Verification items for the finished model (mm, model axes). A direction names the side the tool comes from. Give positions to 0.01 mm unless a question says otherwise; leave off trailing zeros. Order: outer loops, then holes, each group sorted by start corner. A loop starts at its lowest first (then second) coordinate and runs counter-clockwise, first axis right, second up. Notation, with made-up numbers: (82.5, -38) -> (131.5, -38) arc R36 cw to (131.5, -4) -> close; hole circle Ø8 at (-38, 87). An arc over 180 degrees is marked (long way). Return JSON: item names as keys, results as strings. Group by question number.
(1) Cross-section at C-C on z = 4. Enter the section's corners in (x, y), then the cut area to 3 significant figures.
(2) Cross-section at A-A on z = 0. Enter the section's corners in (x, y) (1 decimal).
(3) Depth check by flat-ended pin: pin 1 Ø8.5 at (x, z) = (0, 14.225) entering from +Y; pin 2 Ø6 at (x, y) = (-10, 12) entering from +Z; pin 3 Ø6 at (y, z) = (24, -13.5) entering from -X; pin 4 Ø8 at (y, z) = (4, 10) entering from -X. Enter the tip coordinate at first touch or a pass-through.
(4) Cross-section at D-D on y = 23.5. Enter the section's corners in (x, z) (1 decimal).
(5) Thickness scan on line 1 along Z through (x, y) = (0, 13) (1 decimal); line 2 along X through (y, z) = (20.5, -2); line 3 along Y through (x, z) = (-4.5, 16.5). Record the ranges inside material, lowest first.
(6) Release check for a two-part mould opening along Z. For faces 1 (the face through (6.633, 27.126, -6.083)), 2 (the face through (4, 0, 4)), 3 (the face through (-0.559, 8.874, 11.706)) record: pulls with the +Z half, pulls with the -Z half, needs draft (parallel to the pull), parting line crosses it, or undercut.
(7) Cross-section at B-B on x = 0. Enter the section's corners in (y, z) (1 decimal), then the cut area to 3 significant figures.
(8) Tool access check on faces 4 (the face through (-0.559, 8.874, -16.744)), 5 (the face through (-8.2, 18, -4.5)). Record the directions out of +Z, -Z, +X, -X, +Y, -Y that give a thin tool (end or side, any length) a straight path to the whole face; none if there is none.
from build123d import *

# Parameters (mm, degrees)
CUT_EXTRUDE1_REACH = 46.922
SKETCH2_R          = 4.7625
SKETCH3_R          = 2.58
CUT_EXTRUDE2_DEPTH = 45.92215489


with BuildPart() as part:
    # Sketch1 → Revolve1 (revolve)
    with BuildSketch(Plane.XY, mode=Mode.PRIVATE) as revolve1_sk:
        Polygon((0, 0), (19, 0), (19, 18), (9, 18), (9, 36), (0, 36), align=None)
    revolve(revolve1_sk.sketch.rotate(Axis((0, 36, 0), (0, -1, 0)), 180), axis=Axis((0, 36, 0), (0, -1, 0)))

    # Sketch2 → Cut-Extrude1 (cut, up to next)
    with BuildSketch(Plane.XZ, mode=Mode.PRIVATE) as cut_extrude1_sk1:
        Circle(SKETCH2_R)
    cut_extrude1_tool1 = extrude(cut_extrude1_sk1.sketch, amount=-CUT_EXTRUDE1_REACH, mode=Mode.PRIVATE) & part.part
    add(cut_extrude1_tool1.solids().sort_by_distance((0, 0, 0))[0], mode=Mode.SUBTRACT)

    # Sketch3 → Cut-Extrude2 (cut, through all)
    with BuildSketch(Plane.XZ):
        with Locations((0, 14.225)):
            Circle(SKETCH3_R)
        with Locations((14.225, 0)):
            Circle(SKETCH3_R)
        with Locations((0, -14.225)):
            Circle(SKETCH3_R)
        with Locations((-14.225, 0)):
            Circle(SKETCH3_R)
    extrude(amount=-CUT_EXTRUDE2_DEPTH, mode=Mode.SUBTRACT)


solid = part.part
Verdict:
{
 "1": {"outline": "(-18.57, 0) -> (-2.58, 0) -> (-2.58, 36) -> (-8.06, 36) -> (-8.06, 18) -> (-18.57, 18) -> close; (2.58, 0) -> (18.57, 0) -> (18.57, 18) -> (8.06, 18) -> (8.06, 36) -> (2.58, 36) -> close", "area": "773 mm²"},
 "2": {"outline": "(-19, 0) -> (-16.8, 0) -> (-16.8, 18) -> (-19, 18) -> close; (-11.6, 0) -> (-4.8, 0) -> (-4.8, 36) -> (-9, 36) -> (-9, 18) -> (-11.6, 18) -> close; (4.8, 0) -> (11.6, 0) -> (11.6, 18) -> (9, 18) -> (9, 36) -> (4.8, 36) -> close; (16.8, 0) -> (19, 0) -> (19, 18) -> (16.8, 18) -> close"},
 "3": {"pin 1": "y = 18", "pin 2": "z = 17.66", "pin 3": "through", "pin 4": "x = -18.03"},
 "4": {"outline": "circle Ø18 at (0, 0); hole circle Ø9.5 at (0, 0)"},
 "5": {"line 1": "-19 to -16.8, -11.6 to -4.8, 4.8 to 11.6, 16.8 to 19", "line 2": "-8.77 to -4.32, 4.32 to 8.77", "line 3": "0 to 18"},
 "6": {"face 1": "parting line crosses it", "face 2": "needs draft", "face 3": "undercut"},
 "7": {"outline": "(0, -19) -> (18, -19) -> (18, -16.8) -> (0, -16.8) -> close; (0, -11.6) -> (18, -11.6) -> (18, -9) -> (36, -9) -> (36, -4.8) -> (0, -4.8) -> close; (0, 4.8) -> (36, 4.8) -> (36, 9) -> (18, 9) -> (18, 11.6) -> (0, 11.6) -> close; (0, 16.8) -> (18, 16.8) -> (18, 19) -> (0, 19) -> close", "area": "479 mm²"},
 "8": {"face 4": "+Y, -Y", "face 5": "+Y"}
}
